from build123d import *

# Parameters (mm, degrees)
F0_R     = 3.175
F1_DEPTH = 12.7
F2_SIZE  = 0.79375


with BuildPart() as f1:
    # F0 (on Top) → F1 (new body)
    with BuildSketch(Plane.XY):
        with BuildLine():
            Line((-6.35, 12.7), (-6.35, 26.229805))
            ThreePointArc((-6.35, 26.229805), (-18.492118, 19.656214), (-25.793822, 7.9375))
            Line((-25.793822, 7.9375), (-14.3002, 7.9375))
            ThreePointArc((-14.3002, 7.9375), (-6.3627, 0), (-14.3002, -7.9375))
            Line((-14.3002, -7.9375), (-25.793822, -7.9375))
            ThreePointArc((-25.793822, -7.9375), (-17.284312, -20.726257), (-3.175, -26.800085))
            Line((-3.175, -26.800085), (-3.175, -9.525))
            ThreePointArc((-3.175, -9.525), (0, -6.35), (3.175, -9.525))
            Line((3.175, -9.525), (3.175, -26.800085))
            ThreePointArc((3.175, -26.800085), (18.507165, -19.642047), (26.563956, -4.7625))
            Line((26.563956, -4.7625), (11.1252, -4.7625))
            ThreePointArc((11.1252, -4.7625), (6.3627, 0), (11.1252, 4.7625))
            Line((11.1252, 4.7625), (26.563956, 4.7625))
            ThreePointArc((26.563956, 4.7625), (19.647988, 18.500858), (6.35, 26.229805))
            Line((6.35, 26.229805), (6.35, 12.7))
            ThreePointArc((6.35, 12.7), (0, 6.35), (-6.35, 12.7))
        make_face()
        Circle(F0_R, mode=Mode.SUBTRACT)
    extrude(amount=F1_DEPTH)

    # F2
    f2_edges = [f1.edges().sort_by_distance(p)[0] for p in [
        (-17.284312, -20.726257, 12.7),
        (18.507165, -19.642047, 12.7),
        (19.647988, 18.500858, 12.7),
        (-18.492118, 19.656214, 12.7),
    ]]
    chamfer(f2_edges, length=F2_SIZE)


solid = f1.part
Geometry: final body of the model. Coordinates: model frame, mm. A direction names the side the tool comes from. Coordinates: 2 decimals unless noted, no trailing zeros. Loops run counter-clockwise (first coordinate to the right, second up) from the corner with the lowest first, then second, coordinate; pieces in that order, holes last. Notation, with made-up numbers: (26, 59) - (83, 59) arc R9 ccw to (83, 67) - close; hole circle Ø2 at (65.25, 83). An arc over 180 degrees is marked (long way). Put each result on its own line as item: value. Start each with the question number.
Q1. Set-up query: faces 5 (the flat face through (-3.175, -18, 6)), 6 (the flat face through (19, 4.762, 6)), 7 (the flat face through (-20, 7.938, 6)). Return all of +Z, -Z, +X, -X, +Y, -Y with unobstructed straight access to the full face (end or side cutting, diameter ignored); none if empty.
Q2. Cut plane A-A, the plane y = 0. Return loops of the section in (x, z) (3 decimals), and give its area (3 significant figures).
Q3. Cut plane C-C, the plane x = 0. Return loops of the section in (y, z) (3 decimals).
Q4. Pull-direction query (X, two-part tool) for faces 1 (the conical face through (-17.9, 19.3, 12.57)), 2 (the flat face through (6, 0, 12.7)), 3 (the conical face through (19.31, 17.89, 12.57)), 4 (the cylindrical face through (-0.07, -6.35, 6.26)); classes: released by +X, released by -X, zero draft, split by the parting line, or undercut.
Q5. Line query: line 1 (Y direction, x = 0, z = 5) (3 decimals); line 2 (Y direction, x = 22, z = 4); line 3 (X direction, y = 19.5, z = 3). Output: solid intervals per line, ascending.
Q6. Pin query (flat end, axial travel): pin 1 Ø6 at (y, z) = (-12.5, 5.5) entering from +X; pin 2 Ø2 at (x, z) = (19, 1.5) entering from -Y; pin 3 Ø4 at (y, z) = (17, 9) entering from -X. Return the tip coordinate at first contact, or that it passes through.
Filled sheet:
1. face 5: +Z, -Z, -Y
1. face 6: +Z, -Z, +X
1. face 7: +Z, -Z, -X
2. outline: (-6.363, 0) - (-3.175, 0) - (-3.175, 12.7) - (-6.363, 12.7) - close; (3.175, 0) - (6.363, 0) - (6.363, 12.7) - (3.175, 12.7) - close
2. area: 81.0 mm²
3. outline: (-6.35, 0) - (-3.175, 0) - (-3.175, 12.7) - (-6.35, 12.7) - close; (3.175, 0) - (6.35, 0) - (6.35, 12.7) - (3.175, 12.7) - close
4. face 1: released by -X
4. face 2: zero draft
4. face 3: released by +X
4. face 4: undercut
5. line 1: -6.35 to -3.175, 3.175 to 6.35
5. line 2: -15.63 to -4.76, 4.76 to 15.63
5. line 3: -18.66 to -6.35, 6.35 to 18.66
6. pin 1: x = 25.26
6. pin 2: y = -20.11
6. pin 3: x = -22.43
